Here's how the part is built. I have some questions about the finished solid (model axes, mm). Coordinates: 2 decimals unless noted, no trailing zeros. Write each loop counter-clockwise with the first axis right and the second up, starting at its lowest first coordinate (ties: lowest second). Pieces come first, ordered by that corner, then holes. Notation, with made-up numbers: (66, 60) -> (92, 60) arc R27 ccw to (92, 88) -> close; hole circle Ø3 at (-26, 76). An arc over 180 degrees is marked (long way). Put each result on its own line as item: value.
Autodesk Inventor part; units mm, degrees
ref_plane "YZ Plane" through (0, 0, 0) normal (1, 0, 0) x (0, 1, 0)
ref_plane "XZ Plane" through (0, 0, 0) normal (0, 1, 0) x (-1, 0, 0)
ref_plane "XY Plane" through (0, 0, 0) normal (0, 0, 1) x (1, 0, 0)
sketch "Sketch1" plane through (0, 0, 0) normal (0, 0, 1) x (1, 0, 0)
  line L0 (-546.1, -758.825) -> (546.1, -758.825)
  line L1 (546.1, -758.825) -> (546.1, 758.825)
  line L2 (546.1, 758.825) -> (-546.1, 758.825)
  line L3 (-546.1, 758.825) -> (-546.1, -758.825)
  line L4 (-546.1, -758.825) -> (546.1, 758.825) construction
  line L5 (546.1, -758.825) -> (-546.1, 758.825) construction
  point P0 (0, 0)
  dimension "d0" = 1092.2
  dimension "d1" = 1517.65
extrude "Extrusion1" add sketch "Sketch1" against normal blind 6.35
sketch "Sketch2" plane through (0, 0, 0) normal (0, 0, 1) x (1, 0, 0)
  line L0 (546.1, 758.825) -> (-546.1, 758.825)
  line L1 (-546.1, 758.825) -> (-546.1, -758.825)
  line L2 (-152.4, 352.425) -> (152.4, 352.425)
  line L3 (152.4, 352.425) -> (152.4, 428.625)
  line L4 (152.4, 428.625) -> (-152.4, 428.625)
  line L5 (-152.4, 428.625) -> (-152.4, 352.425)
  line L6 (-152.4, -155.575) -> (152.4, -155.575)
  line L7 (152.4, -155.575) -> (152.4, -79.375)
  line L8 (152.4, -79.375) -> (-152.4, -79.375)
  line L9 (-152.4, -79.375) -> (-152.4, -155.575)
  line L10 (-152.4, -663.575) -> (152.4, -663.575)
  line L11 (152.4, -663.575) -> (152.4, -587.375)
  line L12 (152.4, -587.375) -> (-152.4, -587.375)
  line L13 (-152.4, -587.375) -> (-152.4, -663.575)
  point P0 (0, 0)
  dimension "d4" = 330.2
  dimension "d5" = 406.4
  dimension "d6" = 838.2
  dimension "d7" = 914.4
  dimension "d8" = 1346.2
  dimension "d9" = 1422.4
  dimension "d10" = 393.7
  dimension "d11" = 698.5
extrude "Extrusion2" cut sketch "Sketch2" against normal up to next
sketch "Sketch3" plane through (0, 0, 0) normal (0, 0, 1) x (1, 0, 0)
  line L0 (546.1, 758.825) -> (-546.1, 758.825)
  line L1 (-546.1, 758.825) -> (-546.1, -758.825)
  point P0 (0, 0)
  point P1 (-469.9, 720.725)
  point P2 (-469.9, 530.225)
  point P3 (-469.9, 492.379)
  point P4 (-469.9, -3.175)
  point P5 (-469.9, -41.021)
  point P6 (-469.9, -733.425)
  point P7 (469.9, 720.725)
  point P8 (469.9, 530.225)
  point P9 (469.9, 492.379)
  point P10 (469.9, -3.175)
  point P11 (469.9, -41.021)
  point P12 (469.9, -733.425)
  point P13 (0, -733.425)
  dimension "d14" = 38.1
  dimension "d16" = 1016
  dimension "d17" = 228.6
  dimension "d18" = 266.446
  dimension "d20" = 762
  dimension "d21" = 799.846
  dimension "d22" = 1492.25
  dimension "d23" = 76.2
  dimension "d24" = 1016
  dimension "d32" = 546.1
hole "Hole1" at (-469.9, 720.725, 0) at (-469.9, 530.225, 0) at (-469.9, 492.379, 0) at (-469.9, -3.175, 0) at (-469.9, -41.021, 0) at (-469.9, -733.425, 0) at (469.9, 720.725, 0) at (469.9, 530.225, 0) at (469.9, 492.379, 0) at (469.9, -3.175, 0) at (469.9, -41.021, 0) at (469.9, -733.425, 0) at (0, -733.425, 0) direction (0, 0, -1) diameter 9.652 end through all
properties part number "GE-13010" material "Polycarbonate, Clear"
Item 1: For P1, Ø8.5, axis at x = 469.9, y = -733.425, coming from the -Z side, with a flat end and sliding along its axis, tell me the tip position at first contact or that it passes through.
Output:
P1: passes through
Item 2: Please list where these lines run through material, in increasing order: line 1 along Y through (x, z) = (88.5, -0.5) (3 decimals); line 2 along Y through (x, z) = (0, -1.25) (3 decimals); line 3 along Y through (x, z) = (-3, -1.5) (3 decimals). Write a range as from..to.
Output:
line 1: y = -758.825..-663.575, -587.375..-155.575, -79.375..352.425, 428.625..758.825
line 2: y = -758.825..-738.251, -728.599..-663.575, -587.375..-155.575, -79.375..352.425, 428.625..758.825
line 3: y = -758.825..-737.205, -729.645..-663.575, -587.375..-155.575, -79.375..352.425, 428.625..758.825
Item 3: Imagine slicing it at A-A on z = -1.75. State how many separate pieces and enclosed holes the cut face has, then the cut area to 3 significant figures.
Output:
separate pieces: 1
enclosed holes: 16
area: 1,590,000 mm²
Item 4: Imagine slicing it at B-B on x = -77. Write out the boundary of the cut face in (y, z) (3 decimals), then the cut area to 3 significant figures.
Output:
outline: (-758.825, -6.35) -> (-663.575, -6.35) -> (-663.575, 0) -> (-758.825, 0) -> close; (-587.375, -6.35) -> (-155.575, -6.35) -> (-155.575, 0) -> (-587.375, 0) -> close; (-79.375, -6.35) -> (352.425, -6.35) -> (352.425, 0) -> (-79.375, 0) -> close; (428.625, -6.35) -> (758.825, -6.35) -> (758.825, 0) -> (428.625, 0) -> close
area: 8,190 mm²
